from build123d import *

# Parameters (mm, degrees)
SKETCH1_W                                         = 35
SKETCH1_H                                         = 45
SKETCH1_R                                         = 10
BOSS_EXTRUDE1_DEPTH                               = 30
SKETCH2_W                                         = 54
SKETCH2_H                                         = 80
SKETCH2_R                                         = 2.25
BOSS_EXTRUDE2_DEPTH                               = 20
SKETCH3_W                                         = 40
SKETCH3_H                                         = 80
CUT_EXTRUDE1_DEPTH                                = 10
SKETCH5_W                                         = 40
SKETCH5_H                                         = 30
CUT_EXTRUDE2_DEPTH                                = 10
FILLET1_R                                         = 4
FILLET2_R                                         = 1
CHAMFER1_SIZE                                     = 10
CUT_EXTRUDE3_DEPTH                                = 4
SKETCH11_R                                        = 4
CUT_EXTRUDE4_DEPTH                                = 76.818013919
CUT_EXTRUDE5_DEPTH                                = 94.778592345
CHAMBRAGE_POUR_VIS_SIX_PANS_CREUX_M42_D           = 4.5
CHAMBRAGE_POUR_VIS_SIX_PANS_CREUX_M42_CBORE_D     = 8
CHAMBRAGE_POUR_VIS_SIX_PANS_CREUX_M42_CBORE_DEPTH = 4.4
CHAMBRAGE_POUR_VIS_SIX_PANS_CREUX_M43_D           = 4.5
CHAMBRAGE_POUR_VIS_SIX_PANS_CREUX_M43_CBORE_D     = 8
CHAMBRAGE_POUR_VIS_SIX_PANS_CREUX_M43_CBORE_DEPTH = 4.4


with BuildPart() as part:
    # Sketch1 → Boss-Extrude1 (new body)
    with BuildSketch(Plane.XY):
        Rectangle(SKETCH1_W, SKETCH1_H)
        Circle(SKETCH1_R, mode=Mode.SUBTRACT)
    extrude(amount=BOSS_EXTRUDE1_DEPTH)

    # Sketch2 → Boss-Extrude2 (add)
    with BuildSketch(Plane(origin=(17.5, 0, 0), x_dir=(0, 0, -1), z_dir=(1, 0, 0))):
        with Locations((19.080052459, 0)):
            Rectangle(SKETCH2_W, SKETCH2_H)
        with Locations((-0.419947541, 27.5)):
            Circle(SKETCH2_R, mode=Mode.SUBTRACT)
        with Locations((38.580052459, 27.5)):
            Circle(SKETCH2_R, mode=Mode.SUBTRACT)
        with Locations((38.580052459, -27.5)):
            Circle(SKETCH2_R, mode=Mode.SUBTRACT)
        with Locations((-0.419947541, -27.5)):
            Circle(SKETCH2_R, mode=Mode.SUBTRACT)
    extrude(amount=BOSS_EXTRUDE2_DEPTH)

    # Sketch3 → Cut-Extrude1 (cut)
    with BuildSketch(Plane.ZY.offset(-17.5)):
        with Locations((-26.080052459, 0)):
            Rectangle(SKETCH3_W, SKETCH3_H)
    extrude(amount=-CUT_EXTRUDE1_DEPTH, mode=Mode.SUBTRACT)

    # Sketch5 → Cut-Extrude2 (cut)
    with BuildSketch(Plane(origin=(37.5, 0, 0), x_dir=(0, 0, -1), z_dir=(1, 0, 0))):
        with Locations((26.080052459, 0)):
            Rectangle(SKETCH5_W, SKETCH5_H)
    extrude(amount=-CUT_EXTRUDE2_DEPTH, mode=Mode.SUBTRACT)

    # Fillet1
    fillet1_edges = [part.edges().sort_by_distance(p)[0] for p in [
        (17.5, 0, 7.919947541),
        (17.5, 0, 0),
    ]]
    fillet(fillet1_edges, radius=FILLET1_R)

    # Fillet2
    fillet2_edges = [part.edges().sort_by_distance(p)[0] for p in [
        (17.5, 22.5, 1.95997377),
        (17.5, -22.5, 1.95997377),
        (19.5, 22.5, 7.919947541),
        (19.5, -22.5, 7.919947541),
    ]]
    fillet(fillet2_edges, radius=FILLET2_R)

    # Chamfer1
    chamfer1_edges = [part.edges().sort_by_distance(p)[0] for p in [
        (-17.5, 22.5, 15),
        (-17.5, -22.5, 15),
    ]]
    chamfer(chamfer1_edges, length=CHAMFER1_SIZE)

    # Sketch6 → Cut-Extrude3 (cut)
    with BuildSketch(Plane(origin=(17.5, 0, 0), x_dir=(0, 0, -1), z_dir=(1, 0, 0))):
        Polygon((-18.979274058, -21), (-16.958548116, -17.5), (-18.979274058, -14), (-23.020725942, -14), (-25.041451884, -17.5), (-23.020725942, -21), align=None)
    extrude(amount=-CUT_EXTRUDE3_DEPTH, mode=Mode.SUBTRACT)

    # Sketch10 → Chambrage pour vis à six pans creux M41 (revolve, cut)
    with BuildSketch(Plane(origin=(-7.5, -17.5, 21), x_dir=(0, 0, 1), z_dir=(0, 1, 0))):
        Polygon((0, 0), (0, 45), (2.25, 45), (2.25, 4.4), (4, 4.4), (4, 0), align=None)
    revolve(axis=Axis((-13.85, -17.5, 21), (1, 0, 0)), mode=Mode.SUBTRACT)

    # Sketch11 → Cut-Extrude4 (cut, through all)
    with BuildSketch(Plane(origin=(-7.5, 0, 0), x_dir=(0, 0, -1), z_dir=(1, 0, 0))):
        with Locations(Location((-21, -17.5, 0), (0, 0, 180))):
            Circle(SKETCH11_R)
    extrude(amount=-CUT_EXTRUDE4_DEPTH, mode=Mode.SUBTRACT)

    # Sketch12 → Cut-Extrude5 (cut, through all)
    with BuildSketch(Plane.XY.offset(30)):
        with BuildLine():
            Line((0.75, -9.971835338), (0.75, -31.545013405))
            Line((0.75, -31.545013405), (-0.75, -31.545013405))
            Line((-0.75, -31.545013405), (-0.75, -9.971835338))
            ThreePointArc((-0.75, -9.971835338), (0, -10), (0.75, -9.971835338))
        make_face()
    extrude(amount=-CUT_EXTRUDE5_DEPTH, mode=Mode.SUBTRACT)

    # Chambrage pour vis à six pans creux M42 (through all)
    with Locations(Plane.ZY.offset(-17.5)):
        with Locations((0.419947541, -27.5), (0.419947541, 27.5)):
            CounterBoreHole(CHAMBRAGE_POUR_VIS_SIX_PANS_CREUX_M42_D / 2, CHAMBRAGE_POUR_VIS_SIX_PANS_CREUX_M42_CBORE_D / 2, CHAMBRAGE_POUR_VIS_SIX_PANS_CREUX_M42_CBORE_DEPTH)

    # Chambrage pour vis à six pans creux M43 (through all)
    with Locations(Plane.ZY.offset(-27.5)):
        with Locations((-38.580052459, 27.5), (-38.580052459, -27.5)):
            CounterBoreHole(CHAMBRAGE_POUR_VIS_SIX_PANS_CREUX_M43_D / 2, CHAMBRAGE_POUR_VIS_SIX_PANS_CREUX_M43_CBORE_D / 2, CHAMBRAGE_POUR_VIS_SIX_PANS_CREUX_M43_CBORE_DEPTH)


solid = part.part
CAD build for the part. Positions are in the model's coordinates, mm. A direction names the side the tool comes from. Round coordinates to 2 decimals unless told otherwise and drop trailing zeros. Loops run counter-clockwise (first coordinate to the right, second up) from the corner with the lowest first, then second, coordinate; pieces in that order, holes last.
(1) Cut at B-B (y = -27.5). Give the cut face in (x, z), plus the area to 3 significant figures.
(2) Wall check: line 1 along Y through (x, z) = (35.5, -8.5); line 2 along Z through (x, y) = (32, 27); line 3 along Z through (x, y) = (-12.25, -17.5). Give the ranges that are in metal, low to high.
(3) Cut at D-D (y = -16.5). State how many separate pieces and enclosed holes the cut face has, plus the area to 3 significant figures.
(4) Drop flat-ended pins along their axis: pin 1 (3.5 mm diameter, centred on x = -3, z = 12, fed in from -Y); pin 2 (6 mm diameter, centred on x = 20, y = 23.5, fed in from -Z); pin 3 (8 mm diameter, centred on x = -8.5, y = -13, fed in from -Z). Give the stop position or say it passes through.
(5) Which spindle directions (+Z, -Z, +X, -X, +Y, -Y) get a long thin tool onto all of the face, cutting with end or side? Do faces 1 (the flat face through (-0.75, -16, 15)), 2 (the flat face through (15.5, -19.3, 18)), 3 (the flat face through (31.9, 25.78, -36.86)), 4 (the flat face through (33, 15, -26)). Say none if no direction does.
(6) Two-plate mould, pull along Y, no slides. Class faces 5 (the cylindrical face through (29.6, -29.7, 0.9)), 6 (the flat face through (5, 22.5, 14)), 7 (the flat face through (16, -21, 21)), 8 (the flat face through (0.75, -16, 15)): +Y half, -Y half, draft (parallel to the pull), parting line (faces both ways), or undercut.
(7) Cut at C-C (x = 12). Give the cut face in (y, z), plus the area to 3 significant figures.
(8) Cut at A-A (z = -9.5). Give the cut face in (x, y).
Findings below:
1. outline: (17.5, -6.08) - (27.5, -6.08) - (27.5, -34.58) - (31.9, -34.58) - (31.9, -36.33) - (37.5, -36.33) - (37.5, -1.83) - (21.9, -1.83) - (21.9, -3.58) - (17.5, -3.58) - close; (17.5, 4.42) - (21.9, 4.42) - (21.9, 2.67) - (37.5, 2.67) - (37.5, 7.92) - (17.5, 7.92) - close; (27.5, -46.08) - (37.5, -46.08) - (37.5, -40.83) - (31.9, -40.83) - (31.9, -42.58) - (27.5, -42.58) - close
1. area: 514 mm2
2. line 1: y = -40 to -15, 15 to 40
2. line 2: z = -46.08 to -40.77, -36.39 to -1.77, 2.61 to 7.92
2. line 3: z = 0 to 17, 25 to 30
3. separate pieces: 4
3. enclosed holes: 0
3. area: 1,400 mm2
4. pin 1: stops at y = -22.5
4. pin 2: stops at z = -6.08
4. pin 3: stops at z = 0
5. face 1: +Z, -Z, -Y
5. face 2: +X
5. face 3: -X
5. face 4: -Z, +X, -X
6. face 5: undercut
6. face 6: +Y half
6. face 7: undercut
6. face 8: draft
7. outline: (-22.5, 0) - (22.5, 0) - (22.5, 30) - (-22.5, 30) - close; hole circle Ø4.5 at (-17.5, 21)
7. area: 1,330 mm2
8. outline: (27.5, -40) - (37.5, -40) - (37.5, -15) - (27.5, -15) - close; (27.5, 15) - (37.5, 15) - (37.5, 40) - (27.5, 40) - close
